Source: CAD feature listing. Evaluate the final solid. Frame: model axes, mm. A direction names the side the tool comes from. Round coordinates to 2 decimals unless told otherwise and drop trailing zeros. Write each loop counter-clockwise with the first axis right and the second up, starting at its lowest first coordinate (ties: lowest second). Pieces come first, ordered by that corner, then holes.
Autodesk Inventor part; units mm, degrees
ref_plane "YZ Plane" through (0, 0, 0) normal (1, 0, 0) x (0, 1, 0)
ref_plane "XZ Plane" through (0, 0, 0) normal (0, 1, 0) x (-1, 0, 0)
ref_plane "XY Plane" through (0, 0, 0) normal (0, 0, 1) x (1, 0, 0)
sketch "Sketch1" plane through (0, 0, 0) normal (0, 0, 1) x (1, 0, 0)
  circle A0 centre (-414.4261, -56.251) radius 4.7625
  point P0 (0, 0)
  dimension "d0" = 9.525
extrude "Extrusion1" add sketch "Sketch1" against normal blind 38.1
sketch "Sketch2" plane through (-414.4261, -56.251, 0) normal (0, 0, 1) x (1, 0, 0)
  circle A0 centre (0, 0) radius 4.7625
  line L0 (-8.2489, 0) -> (-4.1244, 7.1437)
  line L1 (-4.1244, 7.1437) -> (4.1244, 7.1438)
  line L2 (4.1244, 7.1438) -> (8.2489, 0)
  line L3 (8.2489, 0) -> (4.1244, -7.1437)
  line L4 (4.1244, -7.1437) -> (-4.1244, -7.1438)
  line L5 (-4.1244, -7.1438) -> (-8.2489, 0)
  point P0 (414.4261, 56.251)
  dimension "d3" = 14.2875
extrude "Extrusion2" add sketch "Sketch2" along normal blind 3.175 contours A0 | L0 L1 L2 L3 L4 L5
thread "Thread1"
chamfer "Chamfer1" distance 0.508 angle 45 1 edges at (-419.1886, -56.251, -38.1)
properties part number "375 bolt x4" material "Steel"
1) Section query B-B on y = -50.5. Return the cut outline in (x, z) (3 decimals), then the cut area to 3 significant figures.
Taken from the geometry:
outline: (-419.355, 0) - (-409.498, 0) - (-409.498, 3.175) - (-419.355, 3.175) - close
area: 31.3 mm2
2) Section query C-C on x = -408.25. Return the cut outline in (y, z) (3 decimals), then the cut area to 3 significant figures.
Taken from the geometry:
outline: (-59.841, 0) - (-52.661, 0) - (-52.661, 3.175) - (-59.841, 3.175) - close
area: 22.8 mm2
3) Material intervals for line 1 (Z direction, x = -419, y = -53.5) (3 decimals); line 2 (X direction, y = -52.5, z = -20.5); line 3 (X direction, y = -53, z = -2), sorted ascending.
Taken from the geometry:
line 1: z = 0 to 3.175
line 2: x = -417.36 to -411.49
line 3: x = -417.91 to -410.95
4) Section query A-A on z = -15.5. Return the cut outline in (x, y) (1 decimal), then the cut area to 3 significant figures.
Taken from the geometry:
outline: circle Ø9.5 at (-414.4, -56.3)
area: 71.3 mm2
5) Reachability of faces 1 (the face through (-415, -51, 0)), 2 (the face through (-415, -56, 3.175)) from +Z, -Z, +X, -X, +Y, -Y: full face, straight path, thin tool, end or side. Return the list, or none.
Taken from the geometry:
face 1: -Z
face 2: +Z, +X, -X, +Y, -Y
6) Contact query for flat-ended pins moving along their axis: P1, Ø3, axis at y = -57, z = -11.5, coming from the +X side; P2, Ø1.5, axis at x = -410, z = -15, coming from the +Y side; P3, Ø6, axis at x = -409.5, z = -30.5, coming from the -Y side. Output: stop coordinate, or through.
Taken from the geometry:
P1: stops at x = -409.66
P2: stops at y = -53.22
P3: stops at y = -60.61
